Source: CAD feature listing. Evaluate the final solid. Frame: model axes, mm. A direction names the side the tool comes from. Give positions to 0.01 mm unless a question says otherwise; leave off trailing zeros. Order: outer loops, then holes, each group sorted by start corner. A loop starts at its lowest first (then second) coordinate and runs counter-clockwise, first axis right, second up.
from build123d import *

# Parameters (mm, degrees)
SKETCH2_R           = 21
BOSS_EXTRUDE1_DEPTH = 33.5
SKETCH3_R           = 2
CUT_EXTRUDE2_DEPTH  = 4
SKETCH4_R           = 2
BOSS_EXTRUDE2_DEPTH = 2.5


with BuildPart() as part:
    # Sketch2 → Boss-Extrude1 (new body)
    with BuildSketch(Plane.XY):
        Circle(SKETCH2_R)
    extrude(amount=-BOSS_EXTRUDE1_DEPTH)

    # Sketch3 → Cut-Extrude2 (cut)
    with BuildSketch(Plane.XY):
        with Locations((0, -15)):
            Circle(SKETCH3_R)
        with Locations((-12.990381057, 7.5)):
            Circle(SKETCH3_R)
        with Locations((12.990381057, 7.5)):
            Circle(SKETCH3_R)
    extrude(amount=-CUT_EXTRUDE2_DEPTH, mode=Mode.SUBTRACT)

    # Sketch4 → Boss-Extrude2 (add)
    with BuildSketch(Plane.XY):
        with Locations((0, 13.5)):
            Circle(SKETCH4_R)
        with Locations((11.691342951, -6.75)):
            Circle(SKETCH4_R)
        with Locations((-11.691342951, -6.75)):
            Circle(SKETCH4_R)
    extrude(amount=BOSS_EXTRUDE2_DEPTH)


solid = part.part
(1) Section A-A, the plane x = 0. Return loops of the section in (y, z).
(2) Section C-C, the plane z = -15. Return loops of the section in (x, y).
(3) Section B-B, the plane y = 7.5. Return loops of the section in (x, z), plus the area to 3 significant figures.
(4) Pin query (flat end, axial travel): pin 1 Ø5 at (x, y) = (-12.99, 7.5) entering from +Z; pin 2 Ø10 at (y, z) = (-10, -11.5) entering from +X; pin 3 Ø4 at (x, z) = (8.5, -30) entering from -Y. Return the tip coordinate at first contact, or that it passes through.
(5) Section D-D, the plane y = 13.5. Return loops of the section in (x, z), plus the area to 3 significant figures.
(6) Access query for faces 5 (the cylindrical face through (20.03, 6.31, -16.52)), 6 (the flat face through (13, 8, -4)). Directions: +Z, -Z, +X, -X, +Y, -Y. A direction counts if a zero-diameter tool reaches every point of the face in a straight line with its end or side. Return the directions, or none.
(7) Draft query along Y for faces 1 (the cylindrical face through (9.693, -6.662, 1.232)), 2 (the cylindrical face through (-11.083, 8.101, -1.972)), 3 (the cylindrical face through (12.73, 9.483, -1.972)), 4 (the flat face through (0, 14, 2.5)). Return one class per face: +Y half, -Y half, draft (parallel to the pull), parting line (faces both ways), or undercut.
(8) Line query: line 1 along Y through (x, z) = (0, -1.9); line 2 along X through (y, z) = (7, -2); line 3 along Z through (x, y) = (3.5, 0). Output: solid intervals per line, ascending.
Checks:
1. outline: (-21, -33.5) - (21, -33.5) - (21, 0) - (15.5, 0) - (15.5, 2.5) - (11.5, 2.5) - (11.5, 0) - (-13, 0) - (-13, -4) - (-17, -4) - (-17, 0) - (-21, 0) - close
2. outline: circle Ø42 at (0, 0)
3. outline: (-19.62, -33.5) - (19.62, -33.5) - (19.62, 0) - (14.99, 0) - (14.99, -4) - (10.99, -4) - (10.99, 0) - (-10.99, 0) - (-10.99, -4) - (-14.99, -4) - (-14.99, 0) - (-19.62, 0) - close
3. area: 1,280 mm2
4. pin 1: stops at z = 0
4. pin 2: stops at x = 20.4
4. pin 3: stops at y = -19.97
5. outline: (-16.09, -33.5) - (16.09, -33.5) - (16.09, 0) - (2, 0) - (2, 2.5) - (-2, 2.5) - (-2, 0) - (-16.09, 0) - close
5. area: 1,090 mm2
6. face 5: +Z, -Z
6. face 6: +Z
7. face 1: parting line
7. face 2: undercut
7. face 3: undercut
7. face 4: draft
8. line 1: y = -21 to -17, -13 to 21
8. line 2: x = -19.8 to -14.93, -11.05 to 11.05, 14.93 to 19.8
8. line 3: z = -33.5 to 0
